Autodesk Inventor part; units mm, degrees
ref_plane "YZ Plane" through (0, 0, 0) normal (1, 0, 0) x (0, 1, 0)
ref_plane "XZ Plane" through (0, 0, 0) normal (0, 1, 0) x (-1, 0, 0)
ref_plane "XY Plane" through (0, 0, 0) normal (0, 0, 1) x (1, 0, 0)
sketch "Sketch1" plane through (0, 0, 0) normal (0, 0, 1) x (1, 0, 0)
  line L0 (0, 0) -> (0, 31.75)
  line L1 (0, 31.75) -> (0.7288, 31.75)
  line L2 (16.4465, 31.75) -> (16.4465, 25.4)
  line L3 (16.4465, 25.4) -> (13.2715, 25.4)
  line L4 (13.2715, 25.4) -> (13.2715, 0)
  line L5 (13.2715, 0) -> (0, 0)
  line L6 (16.4465, 31.75) -> (0.7288, 31.75)
  dimension "d0" = 13.2715
  dimension "d1" = 31.75
  dimension "d2" = 25.4
  dimension "d4" = 3.175
revolve "Revolution1" add sketch "Sketch1" angle 360 about axis through (0, 0, 0) along (0, 1, 0)
sketch "Sketch2" plane through (0, 31.75, 0) normal (0, 1, 0) x (1, 0, 0)
  circle A0 centre (0, 0) radius 6.4135 construction
  line L0 (7.4056, -0.019) -> (3.6864, -6.423)
  line L1 (3.6864, -6.423) -> (-3.7193, -6.404)
  line L2 (-3.7193, -6.404) -> (-7.4056, 0.019)
  line L3 (-7.4056, 0.019) -> (-3.6864, 6.423)
  line L4 (-3.6864, 6.423) -> (3.7193, 6.404)
  line L5 (3.7193, 6.404) -> (7.4056, -0.019)
  point P0 (5.5625, 3.1925)
  dimension "d5" = 12.827
extrude "Extrusion1" cut sketch "Sketch2" against normal through all
properties part number "Climber Axel End Cap"
Read the model definition and answer for the solid it produces. Units are mm, in the model's axes. A direction names the side the tool comes from. Coordinates: 2 decimals unless noted, no trailing zeros. Order: outer loops, then holes, each group sorted by start corner. A loop starts at its lowest first (then second) coordinate and runs counter-clockwise, first axis right, second up. Notation, with made-up numbers: M -31,22.5 L -16,22.5 A23 ccw -16,51.5 Z; hole C 41.5,23.5 d1. An arc over 180 degrees is marked long. Put each result on its own line as item: value. Start each with the question number.
Item 1: Consider probe 1 along X at (y, z) = (5, 0); probe 2 along Z at (x, y) = (0.5, 30); probe 3 along X at (y, z) = (13.5, -6). Determine where each line is inside the solid, lowest interval first. Write a range as [from, to].
Item 2: Section A-A, the plane y = 8 is taken. Determine the outline of the cut face in (x, z).
Item 3: For faces 4 (the face through (5.537, 16.097, -3.237)), 5 (the face through (0, 31.75, 7)), determine the directions among +Z, -Z, +X, -X, +Y, -Y from which every point of the face is accessible in a straight line to the end or side of a thin tool.
Item 4: The mould has two halves that part along X. Classify faces 1 (the face through (-5.57, 16.1, -3.18)), 2 (the face through (1.1, 25.4, -13.5)), 3 (the face through (6.124, 12.522, -11.774)): +X half, -X half, draft (parallel to the pull), parting line (faces both ways), or undercut.
Item 5: Section C-C, the plane z = -4.5 is taken. Determine the outline of the cut face in (x, y).
Item 6: Section D-D, the plane z = -10 is taken. Determine the outline of the cut face in (x, y), plus the area to 3 significant figures.
Item 7: Section B-B, the plane x = 0 is taken. Determine the outline of the cut face in (y, z).
Item 8: Given pin 1 Ø10 at (x, y) = (0, 22.5) entering from -Z; pin 2 Ø1.5 at (x, y) = (3.5, 16) entering from -Z; pin 3 Ø4 at (x, y) = (-6, 5) entering from +Z; pin 4 Ø5 at (x, y) = (2, 5.5) entering from +Z, each flat-ended and moving along its own axis, determine where each tip first touches the part or whether it passes through.
Computed:
1. probe 1: x = [-13.27, -7.39], [7.39, 13.27]
1. probe 2: z = [-16.44, -6.41], [6.41, 16.44]
1. probe 3: x = [-11.84, -3.93], [3.95, 11.84]
2. outline: C 0,0 d26.54; hole M -7.41,-0.02 L -3.69,-6.42 L 3.72,-6.4 L 7.41,0.02 L 3.69,6.42 L -3.72,6.4 Z
3. face 4: +Y, -Y
3. face 5: +Z, -Z, +X, -X, +Y
4. face 1: undercut
4. face 2: draft
4. face 3: parting line
5. outline: M -15.82,25.4 L -12.49,25.4 L -12.49,0 L -4.8,0 L -4.8,31.75 L -15.82,31.75 Z; M 4.81,0 L 12.49,0 L 12.49,25.4 L 15.82,25.4 L 15.82,31.75 L 4.81,31.75 Z
6. outline: M -13.06,25.4 L -8.73,25.4 L -8.73,0 L 8.73,0 L 8.73,25.4 L 13.06,25.4 L 13.06,31.75 L -13.06,31.75 Z
6. area: 609 mm2
7. outline: M 0,-13.27 L 25.4,-13.27 L 25.4,-16.45 L 31.75,-16.45 L 31.75,-6.41 L 0,-6.41 Z; M 0,6.41 L 31.75,6.41 L 31.75,16.45 L 25.4,16.45 L 25.4,13.27 L 0,13.27 Z
8. pin 1: stops at z = -16.45
8. pin 2: stops at z = -12.98
8. pin 3: stops at z = 12.65
8. pin 4: stops at z = 13.27
